```python
from build123d import *

# Parameters (mm, degrees)
BOSS_EXTRU_1_DEPTH      = 20
ESQUISSE2_R             = 1.75
ENL_V_MAT_EXTRU_1_DEPTH = 42.231056256
ESQUISSE3_R             = 1.75
ENL_V_MAT_EXTRU_2_DEPTH = 42.231056256
ESQUISSE4_R             = 1.75
ENL_V_MAT_EXTRU_3_DEPTH = 20


with BuildPart() as part:
    # Esquisse1 → Boss.-Extru.1 (new body)
    with BuildSketch(Plane.XY):
        Polygon((0, 0), (30, 0), (30, 10), (10, 10), (10, 20), (0, 20), align=None)
    extrude(amount=BOSS_EXTRU_1_DEPTH)

    # Esquisse2 → Enlèv. mat.-Extru.1 (cut, through all)
    with BuildSketch(Plane.XZ):
        with Locations(Location((5, 15, 0), (0, 0, 270))):
            Circle(ESQUISSE2_R)
        with Locations(Location((15, 15, 0), (0, 0, 270))):
            Circle(ESQUISSE2_R)
        with Locations(Location((25, 15, 0), (0, 0, 270))):
            Circle(ESQUISSE2_R)
        with Locations(Location((15, 5, 0), (0, 0, 270))):
            Circle(ESQUISSE2_R)
        with Locations(Location((25, 5, 0), (0, 0, 270))):
            Circle(ESQUISSE2_R)
        with Locations(Location((5, 5, 0), (0, 0, 270))):
            Circle(ESQUISSE2_R)
    extrude(amount=-ENL_V_MAT_EXTRU_1_DEPTH, mode=Mode.SUBTRACT)

    # Esquisse3 → Enlèv. mat.-Extru.2 (cut, through all)
    with BuildSketch(Plane.ZY):
        with Locations(Location((15, 5, 0), (0, 0, 180))):
            Circle(ESQUISSE3_R)
        with Locations(Location((5, 5, 0), (0, 0, 180))):
            Circle(ESQUISSE3_R)
        with Locations(Location((5, 15, 0), (0, 0, 270))):
            Circle(ESQUISSE3_R)
        with Locations(Location((15, 15, 0), (0, 0, 270))):
            Circle(ESQUISSE3_R)
    extrude(amount=-ENL_V_MAT_EXTRU_2_DEPTH, mode=Mode.SUBTRACT)

    # Esquisse4 → Enlèv. mat.-Extru.3 (cut)
    with BuildSketch(Plane.XY.offset(20)):
        with Locations((25, 5)):
            Circle(ESQUISSE4_R)
        with Locations(Location((15, 5, 0), (0, 0, 315))):
            Circle(ESQUISSE4_R)
        with Locations(Location((5, 5, 0), (0, 0, 315))):
            Circle(ESQUISSE4_R)
        with Locations((15, 15)):
            Circle(ESQUISSE4_R)
        with Locations(Location((5, 15, 0), (0, 0, 315))):
            Circle(ESQUISSE4_R)
        with Locations((25, 15)):
            Circle(ESQUISSE4_R)
    extrude(amount=-ENL_V_MAT_EXTRU_3_DEPTH, mode=Mode.SUBTRACT)


solid = part.part
```
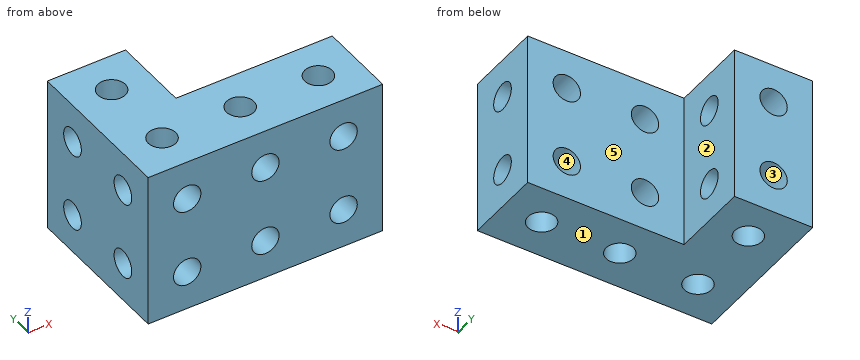
Source: CAD feature listing. Evaluate the final solid. Frame: model axes, mm. Face numbers are marked on the shaded views. A direction names the side the tool comes from. Coordinates: 2 decimals unless noted, no trailing zeros. Loops run counter-clockwise (first coordinate to the right, second up) from the corner with the lowest first, then second, coordinate; pieces in that order, holes last. Notation, with made-up numbers: M 58,16 L 102,16 A20 cw 102,48 Z; hole C -39,35 d8. An arc over 180 degrees is marked long. Use a Markdown table: item, result. Add a question column.
Q1. Draft query along X for the marked faces 1, 2 and 3. Return one class per face: pulls with the +X half, pulls with the -X half, needs draft (parallel to the pull), parting line crosses it, or undercut.
Q2. Section query D-D, the plane y = 1.75. Return loops of the section in (x, z).
Q3. Section query A-A, the plane y = 15. Return loops of the section in (x, z).
Q4. Section query B-B, the plane z = 1.5. Return loops of the section in (x, y), and give its area (3 significant figures).
Q5. Access query for the marked faces 4 and 5. Directions: +Z, -Z, +X, -X, +Y, -Y. A direction counts if a zero-diameter tool reaches every point of the face in a straight line with its end or side. Return the directions, or none.
Q6. Material intervals for L1, parallel to Y at x = 5, z = 1.35; L2, parallel to X at y = 15, z = 19.25, sorted ascending.
Q7. First-contact query: pin 1 (1 mm diameter, centred on x = 23, z = 11.5, fed in from +Y); pin 2 (4.5 mm diameter, centred on y = 15, z = 15, fed in from +X). Flat tips, straight axial feed; report the tip coordinate or a pass-through.
Result:
| question | item | result |
|---|---|---|
| 1 | face 1 | needs draft |
| 1 | face 2 | pulls with the +X half |
| 1 | face 3 | undercut |
| 2 | outline | M 0,0 L 30,0 L 30,20 L 0,20 Z; hole C 5,5 d3.5; hole C 5,15 d3.5; hole C 15,5 d3.5; hole C 15,15 d3.5; hole C 25,5 d3.5; hole C 25,15 d3.5 |
| 3 | outline | M 0,0 L 3.25,0 L 3.25,3.25 L 0,3.25 Z; M 0,6.75 L 3.25,6.75 L 3.25,13.25 L 0,13.25 Z; M 0,16.75 L 3.25,16.75 L 3.25,20 L 0,20 Z; M 6.75,0 L 10,0 L 10,3.25 L 6.75,3.25 Z; M 6.75,6.75 L 10,6.75 L 10,13.25 L 6.75,13.25 Z; M 6.75,16.75 L 10,16.75 L 10,20 L 6.75,20 Z |
| 4 | outline | M 0,0 L 30,0 L 30,10 L 10,10 L 10,20 L 0,20 Z; hole C 5,5 d3.5; hole C 5,15 d3.5; hole C 15,5 d3.5; hole C 25,5 d3.5 |
| 4 | area | 362 mm2 |
| 5 | face 4 | +Y, -Y |
| 5 | face 5 | +Z, -Z, +X, +Y |
| 6 | L1 | y = 0 to 3.25, 6.75 to 13.25, 16.75 to 20 |
| 6 | L2 | x = 0 to 3.25, 6.75 to 10 |
| 7 | pin 1 | stops at y = 10 |
| 7 | pin 2 | stops at x = 10 |
